from build123d import *

# Parameters (mm, degrees)
SKETCH1_R           = 4.0125
SKETCH1_R_2         = 5
SKETCH1_R_3         = 1.8
BOSS_EXTRUDE1_DEPTH = 10


with BuildPart() as part:
    # Sketch1 → Boss-Extrude1 (new body)
    with BuildSketch(Plane.XY):
        with BuildLine():
            Line((-40.735590092, 8.189406634), (-33.201291173, -10))
            Line((-33.201291173, -10), (-9.797958971, -10))
            ThreePointArc((-9.797958971, -10), (0, -14), (9.797958971, -10))
            Line((9.797958971, -10), (33.201291173, -10))
            Line((33.201291173, -10), (40.735590092, 8.189406634))
            ThreePointArc((40.735590092, 8.189406634), (0, 18.25), (-40.735590092, 8.189406634))
        make_face()
        with Locations((20, 0)):
            Circle(SKETCH1_R, mode=Mode.SUBTRACT)
        Circle(SKETCH1_R_2, mode=Mode.SUBTRACT)
        with Locations((-32.07645249, 8.189406634)):
            Circle(SKETCH1_R_3, mode=Mode.SUBTRACT)
        with Locations(Location((32.07645249, 8.189406634, 0), (0, 0, 180))):
            Circle(SKETCH1_R_3, mode=Mode.SUBTRACT)
        Polygon((-25.995276927, 6.573779763), (-35.234072252, 2.746945439), (-31.407237928, -6.491849886), (-22.168442603, -2.665015562), align=None, mode=Mode.SUBTRACT)
    extrude(amount=BOSS_EXTRUDE1_DEPTH)


solid = part.part
Could you check a few things on this model? Use its own coordinates, in mm. A direction names the side the tool comes from. Give positions to 0.01 mm unless a question says otherwise; leave off trailing zeros. Order: outer loops, then holes, each group sorted by start corner. A loop starts at its lowest first (then second) coordinate and runs counter-clockwise, first axis right, second up.
1. Suppose I cut it at A-A (x = 0). List the corners of the cut face in (y, z) for me, plus the area to 4 significant figures.
2. Will these pins go through, and if not, where does the flat tip stop? P1, Ø3, axis at y = 11, z = 5.5, coming from the -X side; P2, Ø4, axis at x = 23.5, z = 1, coming from the +Y side; P3, Ø5, axis at x = -23, z = 3, coming from the -Y side; P4, Ø2, axis at x = 32.08, y = 8.19, coming from the +Z side.
3. Suppose I cut it at B-B (z = 7). Give the number of separate pieces and of enclosed holes in the cut face, plus the area to 3 significant figures.
4. Suppose I cut it at D-D (x = 20). List the corners of the cut face in (y, z) for me.
5. We'd pull the mould along X, two halves only. Please class faces 1 (the cylindrical face through (23.827, 1.205, 4.93)), 2 (the cylindrical face through (0.59, 18.25, 4.93)), 3 (the flat face through (-37.02, -0.78, 4.93)), 4 (the flat face through (-26.853, -4.605, 4.93)): pulls with the +X half, pulls with the -X half, needs draft (parallel to the pull), parting line crosses it, or undercut.
6. Suppose I cut it at C-C (y = 0). List the corners of the cut face in (x, z) for me, plus the area to 3 significant figures.
7. For faces 5 (the flat face through (21, -10, 5)), 6 (the flat face through (-33.347, -1.808, 4.93)), 7 (the flat face through (-1, 6, 0)), 8 (the flat face through (-22, -10, 5)), which set-ups out of +Z, -Z, +X, -X, +Y, -Y let a thin tool reach every point of the face, with its end or its side?
8. I need wall thicknesses on L1, parallel to X at y = -3, z = 1.25; L2, parallel to X at y = 8, z = 7.5; L3, parallel to X at y = -1.5, z = 2.25. Which ranges of each line are inside material? Lowest first, please.
Solved:
1. outline: (-14, 0) - (-5, 0) - (-5, 10) - (-14, 10) - close; (5, 0) - (18.25, 0) - (18.25, 10) - (5, 10) - close
1. area: 222.5 mm2
2. P1: stops at x = -38.14
2. P2: stops at y = 15.57
2. P3: stops at y = -10
2. P4: passes through
3. separate pieces: 1
3. enclosed holes: 5
3. area: 1,700 mm2
4. outline: (-10, 0) - (-4.01, 0) - (-4.01, 10) - (-10, 10) - close; (4.01, 0) - (15.93, 0) - (15.93, 10) - (4.01, 10) - close
5. face 1: undercut
5. face 2: parting line crosses it
5. face 3: pulls with the -X half
5. face 4: undercut
6. outline: (-37.34, 0) - (-34.1, 0) - (-34.1, 10) - (-37.34, 10) - close; (-23.27, 0) - (-5, 0) - (-5, 10) - (-23.27, 10) - close; (5, 0) - (15.99, 0) - (15.99, 10) - (5, 10) - close; (24.01, 0) - (37.34, 0) - (37.34, 10) - (24.01, 10) - close
6. area: 458 mm2
7. face 5: +Z, -Z, +X, -Y
7. face 6: +Z, -Z
7. face 7: -Z, +X, -X, +Y, -Y
7. face 8: +Z, -Z, -X, -Y
8. L1: x = -36.1 to -32.85, -22.98 to -4, 4 to 17.34, 22.66 to 36.1
8. L2: x = -40.66 to -33.87, -30.29 to 30.29, 33.87 to 40.66
8. L3: x = -36.72 to -33.47, -22.65 to -4.77, 4.77 to 16.28, 23.72 to 36.72
